Build history of the part. All positions in model axes, mm. Coordinates: 2 decimals unless noted, no trailing zeros. Order: outer loops, then holes, each group sorted by start corner. A loop starts at its lowest first (then second) coordinate and runs counter-clockwise, first axis right, second up. Notation, with made-up numbers: M 56.5,61.25 L 94.5,61.25 A17 ccw 94.5,80.25 Z; hole C 53,56.5 d2. An arc over 180 degrees is marked long. Write item = value, one per line. Start each with the question number.
Q1. Band-saw the part on A-A on y = -66.15. Write the cut outline in (x, z), plus the area to 3 significant figures.
Q2. Pin check, flat tips, straight feed: P1, Ø1.5, axis at x = -48, z = 1.5, coming from the +Y side; P2, Ø1, axis at y = 13.5, z = 1.5, coming from the -X side; P3, Ø2, axis at x = -18.5, z = 1, coming from the +Y side. Stop position of each tip, or through.
Q3. Pull direction X, two halves, no side cores. Call faces 1 (the face through (-1, 6, 0)), 2 (the face through (-0.25, -75.306, 4.84)), 3 (the face through (-65.09, 37.87, 0.16)): released by +X, released by -X, zero draft, split by the parting line, or undercut.
Q4. Drill centre lines: probe 1 along X at (y, z) = (-0.5, 2.5); probe 2 along Y at (x, z) = (27, 4.15); probe 3 along X at (y, z) = (-7, 3.4). Where is each one in solid material? Low to high.
```python
from build123d import *

# Parameters (mm, degrees)
F1_DEPTH = 5
F2_R     = 5
F3_SIZE  = 1


with BuildPart() as f1:
    # F0 (on Top) → F1 (new body)
    with BuildSketch(Plane.XY):
        with BuildLine():
            ThreePointArc((47.3444830059, 32.0097239742), (49.4933518263, 28.575), (51.3934756327, 24.996663025))
            ThreePointArc((51.3934756327, 24.996663025), (65.9478344982, 38.075), (47.3444830059, 32.0097239742))
        make_face()
        with BuildLine():
            ThreePointArc((4.0489926269, -57.0063869992), (41.8181923846, -38.9533218826), (57.15, 0))
            ThreePointArc((57.15, 0), (55.6922778867, 12.8254701198), (51.3934756327, 24.996663025))
            ThreePointArc((51.3934756327, 24.996663025), (49.4933518263, 28.575), (47.3444830059, 32.0097239742))
            ThreePointArc((47.3444830059, 32.0097239742), (0, 57.15), (-47.3444830059, 32.0097239742))
            ThreePointArc((-47.3444830059, 32.0097239742), (-49.4933518263, 28.575), (-51.3934756327, 24.996663025))
            ThreePointArc((-51.3934756327, 24.996663025), (-49.4933518263, -28.575), (-4.0489926269, -57.0063869992))
            ThreePointArc((-4.0489926269, -57.0063869992), (0, -57.15), (4.0489926269, -57.0063869992))
        make_face()
        with BuildLine():
            ThreePointArc((-51.3934756327, 24.996663025), (-49.4933518263, 28.575), (-47.3444830059, 32.0097239742))
            ThreePointArc((-47.3444830059, 32.0097239742), (-65.9478344982, 38.075), (-51.3934756327, 24.996663025))
        make_face()
        with BuildLine():
            ThreePointArc((-4.0489926269, -57.0063869992), (0, -76.15), (4.0489926269, -57.0063869992))
            ThreePointArc((4.0489926269, -57.0063869992), (0, -57.15), (-4.0489926269, -57.0063869992))
        make_face()
    extrude(amount=F1_DEPTH)

    # F2
    f2_edges = [f1.edges().sort_by_distance(p)[0] for p in [
        (-4.048993, -57.006387, 2.5),
        (-47.344483, 32.009724, 2.5),
        (51.393476, 24.996663, 2.5),
        (47.344483, 32.009724, 2.5),
        (-51.393476, 24.996663, 2.5),
        (4.048993, -57.006387, 2.5),
    ]]
    fillet(f2_edges, radius=F2_R)

    # F3
    f3_edges = [f1.edges().sort_by_distance(p)[0] for p in [
        (65.947834, 38.075, 5),
        (55.195163, 20.905484, 5),
        (45.702262, 37.347671, 5),
        (49.493352, -28.575, 5),
        (0, 57.15, 5),
        (9.492901, -58.253155, 5),
        (-45.702262, 37.347671, 5),
        (0, -76.15, 5),
        (-65.947834, 38.075, 5),
        (-9.492901, -58.253155, 5),
        (-55.195163, 20.905484, 5),
        (-49.493352, -28.575, 5),
        (65.947834, 38.075, 0),
        (55.195163, 20.905484, 0),
        (45.702262, 37.347671, 0),
        (49.493352, -28.575, 0),
        (0, 57.15, 0),
        (9.492901, -58.253155, 0),
        (-45.702262, 37.347671, 0),
        (0, -76.15, 0),
        (-65.947834, 38.075, 0),
        (-9.492901, -58.253155, 0),
        (-55.195163, 20.905484, 0),
        (-49.493352, -28.575, 0),
    ]]
    chamfer(f3_edges, length=F3_SIZE)


solid = f1.part
```
Recorded:
q1.outline = M -10,1 L -9,0 L 9,0 L 10,1 L 10,4 L 9,5 L -9,5 L -10,4 Z
q1.area = 98.0 mm2
q2.P1 = 38.55
q2.P2 = -55.65
q2.P3 = 54.4
q3.face_1 = zero draft
q3.face_2 = split by the parting line
q3.face_3 = undercut
q4.probe_1 = -57.15 to 57.15
q4.probe_2 = -50.2 to 50.2
q4.probe_3 = -56.72 to 56.72
